Source: CAD feature listing. Evaluate the final solid. Frame: model axes, mm. A direction names the side the tool comes from. Coordinates: 2 decimals unless noted, no trailing zeros. Order: outer loops, then holes, each group sorted by start corner. A loop starts at its lowest first (then second) coordinate and runs counter-clockwise, first axis right, second up. Notation, with made-up numbers: (-14, -4.5) - (-9, -4.5) arc R29 ccw to (-9, 31.5) - close; hole circle Ø11 at (60.25, 58). An arc over 180 degrees is marked (long way). One line per question, with ' | ' between items.
from build123d import *

# Parameters (mm, degrees)
F0_W     = 20
F0_H     = 20
F0_W_2   = 17.6
F0_H_2   = 17.6
F1_DEPTH = 10
F2_R     = 1.8
F3_R     = 1.8
F4_R     = 1.8
F5_R     = 1.8
F6_R     = 0.6
F7_R     = 0.6
F8_R     = 0.6
F9_R     = 0.6


with BuildPart() as f1:
    # F0 (on Top) → F1 (new body)
    with BuildSketch(Plane.XY):
        Rectangle(F0_W, F0_H)
        Rectangle(F0_W_2, F0_H_2, mode=Mode.SUBTRACT)
    extrude(amount=F1_DEPTH)

    # F2
    f2_edges = [f1.edges().sort_by_distance(p)[0] for p in [
        (10, -10, 5),
    ]]
    fillet(f2_edges, radius=F2_R)

    # F3
    f3_edges = [f1.edges().sort_by_distance(p)[0] for p in [
        (10, 10, 5),
    ]]
    fillet(f3_edges, radius=F3_R)

    # F4
    f4_edges = [f1.edges().sort_by_distance(p)[0] for p in [
        (-10, 10, 5),
    ]]
    fillet(f4_edges, radius=F4_R)

    # F5
    f5_edges = [f1.edges().sort_by_distance(p)[0] for p in [
        (-10, -10, 5),
    ]]
    fillet(f5_edges, radius=F5_R)

    # F6
    f6_edges = [f1.edges().sort_by_distance(p)[0] for p in [
        (-8.8, 8.8, 5),
    ]]
    fillet(f6_edges, radius=F6_R)

    # F7
    f7_edges = [f1.edges().sort_by_distance(p)[0] for p in [
        (-8.8, -8.8, 5),
    ]]
    fillet(f7_edges, radius=F7_R)

    # F8
    f8_edges = [f1.edges().sort_by_distance(p)[0] for p in [
        (8.8, -8.8, 5),
    ]]
    fillet(f8_edges, radius=F8_R)

    # F9
    f9_edges = [f1.edges().sort_by_distance(p)[0] for p in [
        (8.8, 8.8, 5),
    ]]
    fillet(f9_edges, radius=F9_R)


solid = f1.part
(1) Pull-direction query (X, two-part tool) for faces 1 (the flat face through (0, -8.8, 5)), 2 (the flat face through (0, -10, 5)), 3 (the cylindrical face through (-9.487, -9.459, 5.07)); classes: pulls with the +X half, pulls with the -X half, needs draft (parallel to the pull), parting line crosses it, or undercut.
Taken from the geometry:
face 1: undercut | face 2: needs draft | face 3: pulls with the -X half
(2) Set-up query: faces 4 (the flat face through (10, 0, 5)), 5 (the flat face through (-8.8, 0, 5)). Return all of +Z, -Z, +X, -X, +Y, -Y with unobstructed straight access to the full face (end or side cutting, diameter ignored); none if empty.
Taken from the geometry:
face 4: +Z, -Z, +X, +Y, -Y | face 5: +Z, -Z
(3) Material intervals for L1, parallel to X at y = 2.75, z = 2.25; L2, parallel to X at y = -9, z = 8, sorted ascending. Write a range as from..to.
Taken from the geometry:
L1: x = -10..-8.8, 8.8..10 | L2: x = -9.81..9.81
(4) Cut plane A-A (x = -0.75). Return the cut outline in (y, z).
Taken from the geometry:
outline: (-10, 0) - (-8.8, 0) - (-8.8, 10) - (-10, 10) - close; (8.8, 0) - (10, 0) - (10, 10) - (8.8, 10) - close
(5) Pin query (flat end, axial travel): P1, Ø4, axis at x = 1.5, y = -7.5, coming from the +Z side; P2, Ø4, axis at x = 5, y = 0.5, coming from the -Z side. Return the tip coordinate at first contact, or that it passes through.
Taken from the geometry:
P1: stops at z = 10 | P2: passes through
(6) Cut plane C-C (z = 1.25). Return the cut outline in (x, y), and give its area (3 significant figures).
Taken from the geometry:
outline: (-10, -8.2) arc R1.8 ccw to (-8.2, -10) - (8.2, -10) arc R1.8 ccw to (10, -8.2) - (10, 8.2) arc R1.8 ccw to (8.2, 10) - (-8.2, 10) arc R1.8 ccw to (-10, 8.2) - close; hole (-8.8, -8.2) arc R0.6 ccw to (-8.2, -8.8) - (8.2, -8.8) arc R0.6 ccw to (8.8, -8.2) - (8.8, 8.2) arc R0.6 ccw to (8.2, 8.8) - (-8.2, 8.8) arc R0.6 ccw to (-8.8, 8.2) - close | area: 87.8 mm²
